from build123d import *

# Parameters (mm, degrees)
F0_W     = 15
F0_H     = 15
F1_DEPTH = 8
F2_W     = 15
F2_H     = 4.8
F3_DEPTH = 5
F4_R     = 2.5
F5_R     = 2.5


with BuildPart() as f1:
    # F0 (on Top) → F1 (new body)
    with BuildSketch(Plane.XY):
        with Locations((-7.5, 0)):
            Rectangle(F0_W, F0_H)
    extrude(amount=F1_DEPTH)

    # F2 (on face) → F3 (cut)
    with BuildSketch(Plane(origin=(-15, 0, 0), x_dir=(0, -1, 0), z_dir=(-1, 0, 0))):
        with Locations((0, 4.1)):
            Rectangle(F2_W, F2_H)
    extrude(amount=-F3_DEPTH, mode=Mode.SUBTRACT)

    # F4
    f4_edges = [f1.edges().sort_by_distance(p)[0] for p in [
        (0, -7.5, 4),
        (0, 7.5, 4),
    ]]
    fillet(f4_edges, radius=F4_R)

    # F5
    f5_edges = [f1.edges().sort_by_distance(p)[0] for p in [
        (-15, -7.5, 0.85),
        (-15, -7.5, 7.25),
        (-15, 7.5, 0.85),
        (-15, 7.5, 7.25),
    ]]
    fillet(f5_edges, radius=F5_R)


solid = f1.part
For this review, take the finished solid that the model builds, in its own axes (mm). A direction names the side the tool comes from. Give positions to 0.01 mm unless a question says otherwise; leave off trailing zeros. Order: outer loops, then holes, each group sorted by start corner. A loop starts at its lowest first (then second) coordinate and runs counter-clockwise, first axis right, second up. Notation, with made-up numbers: (26.25, 19.25) - (43.25, 19.25) arc R15 cw to (43.25, 45.25) - close; hole circle Ø4 at (23, 0.25). An arc over 180 degrees is marked (long way). Answer as a JSON object with one key per item and string values. Group by question number.
Item 1: Take a section at A-A on y = 0.75. Give the boundary of the cut face in (x, z).
Item 2: Take a section at B-B on z = 5.75. Give the boundary of the cut face in (x, y).
Item 3: Take a section at D-D on x = -1.75. Give the boundary of the cut face in (y, z), and give its area (3 significant figures).
Item 4: Clearance check with a flat-ended pin moving along its axis: pin 1 Ø2.5 at (y, z) = (3, 4.5) entering from -X. State where the tip first meets the part, or that it passes through.
Item 5: Machinability: for faces 4 (the flat face through (-13, 0, 1.7)), 5 (the cylindrical face through (-14, -7, 1)), which of the approach directions +Z, -Z, +X, -X, +Y, -Y give a long, thin tool a straight path to every point of the face, cutting with its end or side? Answer none if there is none.
Item 6: Draft analysis for pull direction Z (two halves, no side actions). For faces 1 (the cylindrical face through (-14, 7, 7)), 2 (the flat face through (-10, 0, 4)), 3 (the flat face through (-8, 0, 8)), state which applies: pulls with the +Z half, pulls with the -Z half, needs draft (parallel to the pull), parting line crosses it, or undercut.
Item 7: Take a section at C-C on z = 1. Give the boundary of the cut face in (x, y), and give its area (3 significant figures).
Item 8: Wall thickness on line 1 along Z through (x, y) = (-11, 5.25); line 2 along X through (y, z) = (-4.5, 1.75); line 3 along Y through (x, z) = (-13.5, 1.5): over which ranges is each line inside the solid? List them lowest first.
Reported:
{
 "1": {"outline": "(-15, 0) - (0, 0) - (0, 8) - (-15, 8) - (-15, 6.5) - (-10, 6.5) - (-10, 1.7) - (-15, 1.7) - close"},
 "2": {"outline": "(-10, -7.5) - (-2.5, -7.5) arc R2.5 ccw to (0, -5) - (0, 5) arc R2.5 ccw to (-2.5, 7.5) - (-10, 7.5) - close"},
 "3": {"outline": "(-7.38, 0) - (7.38, 0) - (7.38, 8) - (-7.38, 8) - close", "area": "118 mm^2"},
 "4": {"pin 1": "x = -10"},
 "5": {"face 4": "-X, +Y, -Y", "face 5": "+Z, -Z, -X, -Y"},
 "6": {"face 1": "needs draft", "face 2": "undercut", "face 3": "pulls with the +Z half"},
 "7": {"outline": "(-15, -5) arc R2.5 ccw to (-12.5, -7.5) - (-2.5, -7.5) arc R2.5 ccw to (0, -5) - (0, 5) arc R2.5 ccw to (-2.5, 7.5) - (-12.5, 7.5) arc R2.5 ccw to (-15, 5) - close", "area": "220 mm^2"},
 "8": {"line 1": "0 to 1.7, 6.5 to 8", "line 2": "-10 to 0", "line 3": "-7.29 to 7.29"}
}
